Print and shaded views of the part. All mm, measured from the part's lowest x, y and z. A direction names the side the tool comes from. Coordinates: 2 decimals unless noted, no trailing zeros. Loops run counter-clockwise (first coordinate to the right, second up) from the corner with the lowest first, then second, coordinate; pieces in that order, holes last. Notation, with made-up numbers: (-17, -13.75) -> (29, -13.75) arc R27 cw to (29, 12.25) -> close; hole circle Ø8 at (80.25, 83). An arc over 180 degrees is marked (long way). One line per question, with ' | ' between items. Start each with the question number.
1) Cut at A-A (x = 81.09). List the corners of the cut face in (y, z), plus the area to 3 significant figures.
2) Cut at C-C (z = 16.25). List the corners of the cut face in (x, y), plus the area to 3 significant figures.
3) Probe L1, parallel to X at y = 75.6, z = 4.75; L2, parallel to Y at x = 10.5, z = 5.25; L3, parallel to Z at x = 1, y = 45. List the from-to ranges inside material, lowest first. Write a range as from..to.
4) Cut at B-B (y = 75.6). List the corners of the cut face in (x, z), plus the area to 3 significant figures.
5) Drop flat-ended pins along their axis: pin 1 (1.5 mm diameter, centred on x = 18.5, y = 64, fed in from +Z); pin 2 (12 mm diameter, centred on x = 55, z = 19, fed in from -Y); pin 3 (1 mm diameter, centred on x = 18, z = 12, fed in from +Y); pin 4 (1.5 mm diameter, centred on x = 45, y = 69.5, fed in from -Z). Give the stop position or say it passes through.
6) Cut at D-D (x = 10.5). List the corners of the cut face in (y, z), plus the area to 3 significant figures.
7) 3-axis set-ups, long thin cutter, end or side, ignore diameter. For the marked faces 1, 2, 3 and 4: which of +Z, -Z, +X, -X, +Y, -Y reach the whole face in a straight line?
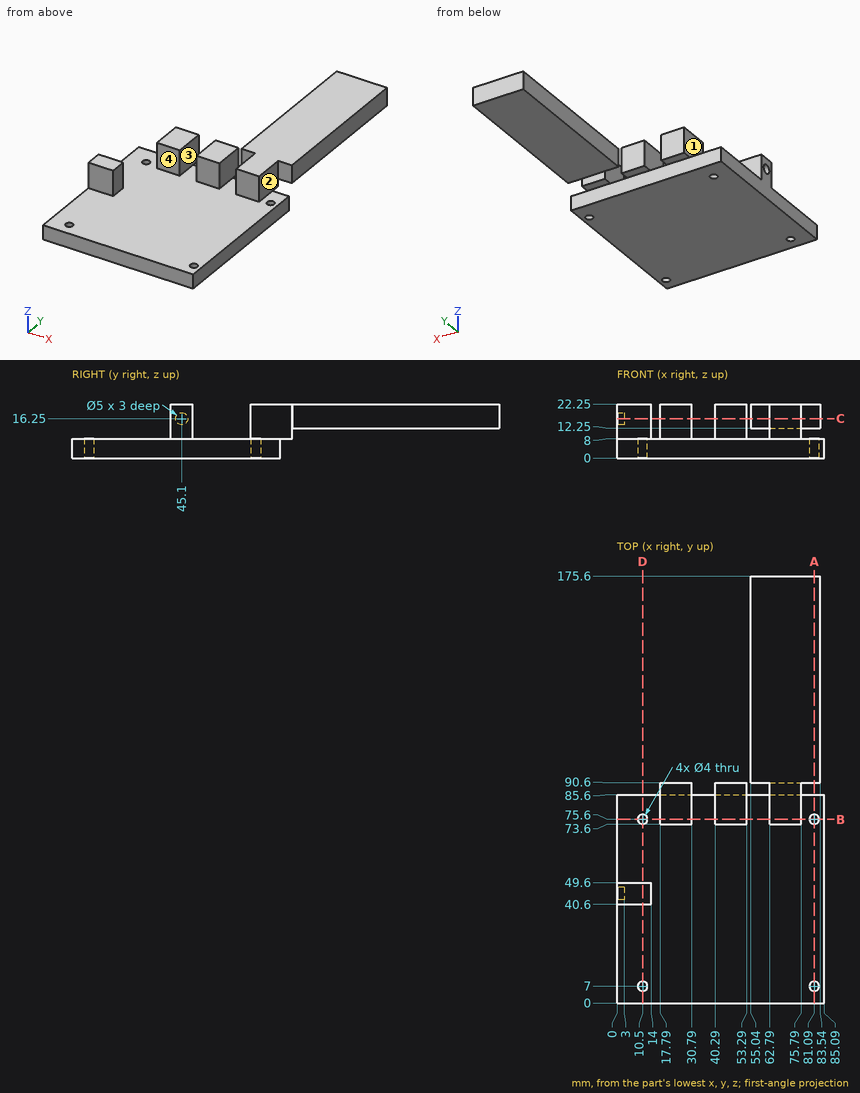
Reported:
1) outline: (0, 0) -> (5, 0) -> (5, 8) -> (0, 8) -> close; (9, 0) -> (73.6, 0) -> (73.6, 8) -> (9, 8) -> close; (77.6, 0) -> (85.6, 0) -> (85.6, 8) -> (77.6, 8) -> close; (90.6, 12.25) -> (175.6, 12.25) -> (175.6, 22.25) -> (90.6, 22.25) -> close | area: 1,470 mm²
2) outline: (0, 40.6) -> (14, 40.6) -> (14, 49.6) -> (0, 49.6) -> (0, 47.6) -> (3, 47.6) -> (3, 42.6) -> (0, 42.6) -> close; (17.79, 73.6) -> (30.79, 73.6) -> (30.79, 90.6) -> (17.79, 90.6) -> close; (40.29, 73.6) -> (53.29, 73.6) -> (53.29, 90.6) -> (40.29, 90.6) -> close; (55.04, 90.6) -> (62.79, 90.6) -> (62.79, 73.6) -> (75.79, 73.6) -> (75.79, 90.6) -> (83.54, 90.6) -> (83.54, 175.6) -> (55.04, 175.6) -> close | area: 3,200 mm²
3) L1: x = 0..8.5, 12.5..79.09, 83.09..85.09 | L2: y = 0..5, 9..73.6, 77.6..85.6 | L3: z = 0..13.75, 18.75..22.25
4) outline: (0, 0) -> (8.5, 0) -> (8.5, 8) -> (0, 8) -> close; (12.5, 0) -> (79.09, 0) -> (79.09, 8) -> (75.79, 8) -> (75.79, 22.25) -> (62.79, 22.25) -> (62.79, 8) -> (53.29, 8) -> (53.29, 22.25) -> (40.29, 22.25) -> (40.29, 8) -> (30.79, 8) -> (30.79, 22.25) -> (17.79, 22.25) -> (17.79, 8) -> (12.5, 8) -> close; (83.09, 0) -> (85.09, 0) -> (85.09, 8) -> (83.09, 8) -> close | area: 1,170 mm²
5) pin 1: stops at z = 8 | pin 2: stops at y = 73.6 | pin 3: stops at y = 90.6 | pin 4: stops at z = 0
6) outline: (0, 0) -> (5, 0) -> (5, 8) -> (0, 8) -> close; (9, 0) -> (73.6, 0) -> (73.6, 8) -> (49.6, 8) -> (49.6, 22.25) -> (40.6, 22.25) -> (40.6, 8) -> (9, 8) -> close; (77.6, 0) -> (85.6, 0) -> (85.6, 8) -> (77.6, 8) -> close | area: 749 mm²
7) face 1: +Z, -X, +Y, -Y | face 2: +Z, +X, -Y | face 3: +Z, +Y, -Y | face 4: +Z, +X, -X, -Y
